from build123d import *

# Parameters (mm, degrees)
SKETCH1_R           = 1
BOSS_EXTRUDE1_DEPTH = 2.5
SKETCH2_R           = 3.35
CUT_EXTRUDE1_DEPTH  = 2.3
CHAMFER1_SIZE       = 0.7
CHAMFER1_SIZE2      = 1.923234194
CHAMFER2_SIZE       = 0.3
CHAMFER2_SIZE2      = 1.119615242
CHAMFER3_SIZE       = 0.3
CHAMFER3_SIZE2      = 0.519615242
SKETCH3_R           = 2
CUT_EXTRUDE2_DEPTH  = 10


with BuildPart() as part:
    # Sketch1 → Boss-Extrude1 (new body)
    with BuildSketch(Plane.XY):
        with BuildLine():
            Line((-8.251445087, 2.384393064), (-3.005780347, 4.037572254))
            ThreePointArc((-3.005780347, 4.037572254), (0, 4.5), (3.005780347, 4.037572254))
            Line((3.005780347, 4.037572254), (8.251445087, 2.384393064))
            ThreePointArc((8.251445087, 2.384393064), (10, 0), (8.251445087, -2.384393064))
            Line((8.251445087, -2.384393064), (3.005780347, -4.037572254))
            ThreePointArc((3.005780347, -4.037572254), (0, -4.5), (-3.005780347, -4.037572254))
            Line((-3.005780347, -4.037572254), (-8.251445087, -2.384393064))
            ThreePointArc((-8.251445087, -2.384393064), (-10, 0), (-8.251445087, 2.384393064))
        make_face()
        with Locations((7.5, 0)):
            Circle(SKETCH1_R, mode=Mode.SUBTRACT)
        with Locations((-7.5, 0)):
            Circle(SKETCH1_R, mode=Mode.SUBTRACT)
    extrude(amount=BOSS_EXTRUDE1_DEPTH)

    # Sketch2 → Cut-Extrude1 (cut)
    with BuildSketch(Plane.XY.offset(2.5)):
        Circle(SKETCH2_R)
    extrude(amount=-CUT_EXTRUDE1_DEPTH, mode=Mode.SUBTRACT)

    # Chamfer1
    chamfer1_edges = [part.edges().sort_by_distance(p)[0] for p in [
        (-5.628612717, -3.210982659, 0),
        (-10, 0, 0),
        (-5.628612717, 3.210982659, 0),
        (0, 4.5, 0),
        (5.628612717, 3.210982659, 0),
        (10, 0, 0),
        (5.628612717, -3.210982659, 0),
        (0, -4.5, 0),
    ]]
    chamfer1_side = [part.faces().sort_by_distance(p)[0] for p in [
        (0, 0, 0),
    ]]
    chamfer(chamfer1_edges, length=CHAMFER1_SIZE, length2=CHAMFER1_SIZE2, reference=chamfer1_side[0])

    # Chamfer2
    chamfer2_edges = [part.edges().sort_by_distance(p)[0] for p in [
        (-3.35, 0, 2.5),
    ]]
    chamfer2_side = [part.faces().sort_by_distance(p)[0] for p in [
        (-5.562690807, -3.001807369, 2.5),
    ]]
    chamfer(chamfer2_edges, length=CHAMFER2_SIZE, length2=CHAMFER2_SIZE2, reference=chamfer2_side[0])

    # Chamfer3
    chamfer3_edges = [part.edges().sort_by_distance(p)[0] for p in [
        (6.5, 0, 2.5),
        (-8.5, 0, 2.5),
    ]]
    chamfer3_side = [part.faces().sort_by_distance(p)[0] for p in [
        (-3.869317122, 0, 2.5),
    ]]
    chamfer(chamfer3_edges, length=CHAMFER3_SIZE, length2=CHAMFER3_SIZE2, reference=chamfer3_side[0])

    # Sketch3 → Cut-Extrude2 (cut)
    with BuildSketch(Plane.XY.offset(0.2)):
        Circle(SKETCH3_R)
    extrude(amount=-CUT_EXTRUDE2_DEPTH, mode=Mode.SUBTRACT)


solid = part.part
Could you check a few things on this model? Use its own coordinates, in mm. A direction names the side the tool comes from. Give positions to 0.01 mm unless a question says otherwise; leave off trailing zeros. Order: outer loops, then holes, each group sorted by start corner. A loop starts at its lowest first (then second) coordinate and runs counter-clockwise, first axis right, second up. Notation, with made-up numbers: (21, -25.5) -> (48, -25.5) arc R13 ccw to (48, -17.5) -> close; hole circle Ø4 at (45, -33). An arc over 180 degrees is marked (long way). Answer in a Markdown table with one row per item. Add a question column.
Item 1: Imagine slicing it at A-A (y = 0). List the corners of the cut face in (x, z) for me, and give its area (3 significant figures).
Item 2: Imagine slicing it at D-D (x = -7.5). List the corners of the cut face in (y, z) for me.
Item 3: Please list where these lines run through material, in increasing order: probe 1 along Y at (x, z) = (0, 0.1); probe 2 along X at (y, z) = (0.5, 0.45); probe 3 along Y at (x, z) = (2, 1.1).
Item 4: I'm going to push a flat-ended pin straight in: P1, Ø2, axis at x = -1, y = 1, coming from the +Z side. Where does the tip first touch, or does it pass through?
Item 5: For faces 1 (the flat face through (0, -2.2, 0.2)), 2 (the flat face through (-2, -1, 0)), which set-ups out of +Z, -Z, +X, -X, +Y, -Y let a thin tool reach every point of the face, with its end or its side?
Item 6: Imagine slicing it at C-C (z = 0.8). List the corners of the cut face in (x, y) for me, and give its area (3 significant figures).
Item 7: We'd pull the mould along X, two halves only. Please class faces 3 (the cylindrical face through (-3.347, 0.147, 0.798)), 4 (the conical face through (-9.577, -0.037, 0.761)), 5 (the flat face through (5.5, 2.9, 1)): pulls with the +X half, pulls with the -X half, needs draft (parallel to the pull), parting line crosses it, or undercut.
Item 8: Imagine slicing it at B-B (x = 0). List the corners of the cut face in (y, z) for me, and give its area (3 significant figures).
Result:
| question | item | result |
|---|---|---|
| 1 | outline | (-10, 1.92) -> (-9.3, 0) -> (-8.5, 0) -> (-8.5, 1.98) -> (-8.8, 2.5) -> (-10, 2.5) -> close; (-6.5, 0) -> (-2, 0) -> (-2, 0.2) -> (-3.35, 0.2) -> (-3.35, 1.38) -> (-3.65, 2.5) -> (-6.2, 2.5) -> (-6.5, 1.98) -> close; (2, 0) -> (6.5, 0) -> (6.5, 1.98) -> (6.2, 2.5) -> (3.65, 2.5) -> (3.35, 1.38) -> (3.35, 0.2) -> (2, 0.2) -> close; (8.5, 0) -> (9.3, 0) -> (10, 1.92) -> (10, 2.5) -> (8.8, 2.5) -> (8.5, 1.98) -> close |
| 1 | area | 21.8 mm2 |
| 2 | outline | (-2.62, 1.92) -> (-1.89, 0) -> (-1, 0) -> (-1, 1.98) -> (-1.3, 2.5) -> (-2.62, 2.5) -> close; (1, 0) -> (1.89, 0) -> (2.62, 1.92) -> (2.62, 2.5) -> (1.3, 2.5) -> (1, 1.98) -> close |
| 3 | probe 1 | -3.84 to -2, 2 to 3.84 |
| 3 | probe 2 | -9.4 to -8.37, -6.63 to -3.31, 3.31 to 6.63, 8.37 to 9.4 |
| 3 | probe 3 | -3.99 to -2.69, 2.69 to 3.99 |
| 4 | P1 | z = 0.2 |
| 5 | face 1 | +Z |
| 5 | face 2 | -Z, +X, -X, +Y, -Y |
| 6 | outline | (-8.13, -1.99) -> (-2.88, -3.65) arc R9.59 ccw to (2.88, -3.65) -> (8.13, -1.99) arc R2.09 ccw to (8.13, 1.99) -> (2.88, 3.65) arc R9.59 ccw to (-2.88, 3.65) -> (-8.13, 1.99) arc R2.09 ccw to start; hole circle Ø2 at (-7.5, 0); hole circle Ø6.7 at (0, 0); hole circle Ø2 at (7.5, 0) |
| 6 | area | 71.7 mm2 |
| 7 | face 3 | undercut |
| 7 | face 4 | pulls with the -X half |
| 7 | face 5 | pulls with the +X half |
| 8 | outline | (-4.5, 1.92) -> (-3.8, 0) -> (-2, 0) -> (-2, 0.2) -> (-3.35, 0.2) -> (-3.35, 1.38) -> (-3.65, 2.5) -> (-4.5, 2.5) -> close; (2, 0) -> (3.8, 0) -> (4.5, 1.92) -> (4.5, 2.5) -> (3.65, 2.5) -> (3.35, 1.38) -> (3.35, 0.2) -> (2, 0.2) -> close |
| 8 | area | 4.61 mm2 |
